Work out the finished part from the listing and answer in its coordinate system (mm). A direction names the side the tool comes from. Round coordinates to 2 decimals unless told otherwise and drop trailing zeros. Write each loop counter-clockwise with the first axis right and the second up, starting at its lowest first coordinate (ties: lowest second). Pieces come first, ordered by that corner, then holes. Notation, with made-up numbers: M 50,40 L 67,40 A11 cw 67,58 Z; hole C 57,19.25 d1. An arc over 180 degrees is marked long. One line per item, written item: value. Start each with the question number.
Q1. Find section B-B (y = 0). Write down the section's boundary in (x, z), and give its area (3 significant figures).
Q2. Given pin 1 Ø1.8 at (x, y) = (-10.25, 2.83) entering from -Z; pin 2 Ø7 at (x, y) = (0, 0) entering from -Z, each flat-ended and moving along its own axis, determine where each tip first touches the part or whether it passes through.
Q3. The mould has two halves that part along Y. Classify faces 3 (the cylindrical face through (-3.01, -8.76, 0.51)), 4 (the flat face through (-0.2, -3.1, 0)), 5 (the cylindrical face through (-14.985, 0.66, 0.496)): released by +Y, released by -Y, zero draft, split by the parting line, or undercut.
Q4. Consider probe 1 along Y at (x, z) = (10.25, 0.6) (3 decimals); probe 2 along X at (y, z) = (3, 0.3); probe 3 along Y at (x, z) = (10.5, 0.2). Determine where each line is inside the solid, lowest interval first.
Q5. Find section A-A (x = 0). Write down the section's boundary in (y, z).
Q6. Find section C-C (z = 0.55). Count the separate pieces of the cut face and the enclosed holes in it, and give its area (3 significant figures).
Q7. A tool of negligible diameter and unlimited length cuts with its end or side. For faces 1 (the flat face through (-0.1, 5.751, 0.6)), 2 (the cylindrical face through (9.5, -2.2, 0.5)), from which of +Z, -Z, +X, -X, +Y, -Y can it reach the whole face along a straight path? Write none if from no direction.
from build123d import *

# Parameters (mm, degrees)
F0_R     = 15
F1_DEPTH = 1
F2_W     = 12.5
F2_H     = 11.5
F3_DEPTH = 0.85
F5_R     = 2.950818
F6_DEPTH = 0.15
F7_R     = 0.25
F8_R     = 1
F9_DEPTH = 1


with BuildPart() as f1:
    # F0 (on Top) → F1 (new body)
    with BuildSketch(Plane.XY):
        Circle(F0_R)
    extrude(amount=F1_DEPTH)

    # F2 (on face) → F3 (cut)
    with BuildSketch(Plane.XY.offset(1)):
        with Locations((0, 0.000526)):
            Rectangle(F2_W, F2_H)
    extrude(amount=-F3_DEPTH, mode=Mode.SUBTRACT)

    # F5 (on offset) → F6 (cut)
    with BuildSketch(Plane.XY.offset(0.15)):
        Circle(F5_R)
    extrude(amount=-F6_DEPTH, mode=Mode.SUBTRACT)

    # F7
    f7_edges = [f1.edges().sort_by_distance(p)[0] for p in [
        (-15, 0, 1),
        (-15, 0, 0),
    ]]
    fillet(f7_edges, radius=F7_R)

    # F8 (on face) → F9 (cut)
    with BuildSketch(Plane.XY.offset(1)):
        with Locations((-10.25, 2.832073)):
            Circle(F8_R)
        with Locations((-10.25, -2.917927)):
            Circle(F8_R)
        with Locations((-2.875, 9.750526)):
            Circle(F8_R)
        with Locations((2.875, 9.750526)):
            Circle(F8_R)
        with Locations((10.25, 2.875)):
            Circle(F8_R)
        with Locations((10.25, -2.863999)):
            Circle(F8_R)
        with Locations((2.875, -9.749474)):
            Circle(F8_R)
        with Locations((-2.875, -9.749474)):
            Circle(F8_R)
    extrude(amount=-F9_DEPTH, mode=Mode.SUBTRACT)


solid = f1.part
The answers:
1. outline: M -15,0.25 A0.25 ccw -14.75,0 L -2.95,0 L -2.95,0.15 L -6.25,0.15 L -6.25,1 L -14.75,1 A0.25 ccw -15,0.75 Z; M 2.95,0 L 14.75,0 A0.25 ccw 15,0.25 L 15,0.75 A0.25 ccw 14.75,1 L 6.25,1 L 6.25,0.15 L 2.95,0.15 Z
1. area: 18.4 mm2
2. pin 1: through
2. pin 2: z = 0
3. face 3: undercut
3. face 4: zero draft
3. face 5: split by the parting line
4. probe 1: -10.952 to -3.864, -1.864 to 1.875, 3.875 to 10.952
4. probe 2: -14.7 to -11.24, -9.26 to -6.25, 6.25 to 9.26, 11.24 to 14.7
4. probe 3: -10.71 to -3.83, -1.9 to 1.91, 3.84 to 10.71
5. outline: M -15,0.25 A0.25 ccw -14.75,0 L -2.95,0 L -2.95,0.15 L -5.75,0.15 L -5.75,1 L -14.75,1 A0.25 ccw -15,0.75 Z; M 2.95,0 L 14.75,0 A0.25 ccw 15,0.25 L 15,0.75 A0.25 ccw 14.75,1 L 5.75,1 L 5.75,0.15 L 2.95,0.15 Z
6. separate pieces: 1
6. enclosed holes: 9
6. area: 538 mm2
7. face 1: +Z
7. face 2: +Z, -Z
